Design review of the part shown in the three views and the two pictorial views. Dimensions are in mm from the part's minimum x, y and z. A direction names the side the tool comes from. Give positions to 0.01 mm unless a question says otherwise; leave off trailing zeros. Write each loop counter-clockwise with the first axis right and the second up, starting at its lowest first coordinate (ties: lowest second). Pieces come first, ordered by that corner, then holes. Notation, with made-up numbers: M 11,21.25 L 36,21.25 A25 cw 36,52.25 Z; hole C 71,-36.75 d10. An arc over 180 degrees is marked long. Use one line per item in the form item = value. Start each with the question number.
Q1. Consider section D-D on x = 13.5. Write out the cut boundary in (y, z), and give its area (3 significant figures).
Q2. Consider section B-B on z = 3.35. Write out the cut boundary in (x, y), and give its area (4 significant figures).
Q3. For probe 1 along X at (y, z) = (2.5, 1.2); probe 2 along Y at (x, z) = (16.5, 3.8), list the stretches that pass through material, from the lowest coordinate up. Write a range as [from, to].
Q4. Consider section C-C on y = 17.5. Write out the cut boundary in (x, z).
Q5. Consider section A-A on x = 3.75. Write out the cut boundary in (y, z), and give its area (3 significant figures).
Q6. Mouldability with a two-part tool opening along X and no side actions: class the marked faces 1, 2 and 3 as released by +X, released by -X, zero draft, split by the parting line, or undercut.
Q7. Clearance check with flat-ended pins moving along their axes: pin 1 Ø2 at (y, z) = (2.5, 2.5) entering from -X; pin 2 Ø2.5 at (x, z) = (2.5, 2.5) entering from -Y; pin 3 Ø8 at (x, y) = (8, 9) entering from -Z. State where each tip first meets the part, or that it passes through.
Q8. Tool access review of the marked faces 4, 5, 6 and 7: name each direction out of +Z, -Z, +X, -X, +Y, -Y from which nothing blocks a thin tool from reaching the whole face with its end or side.
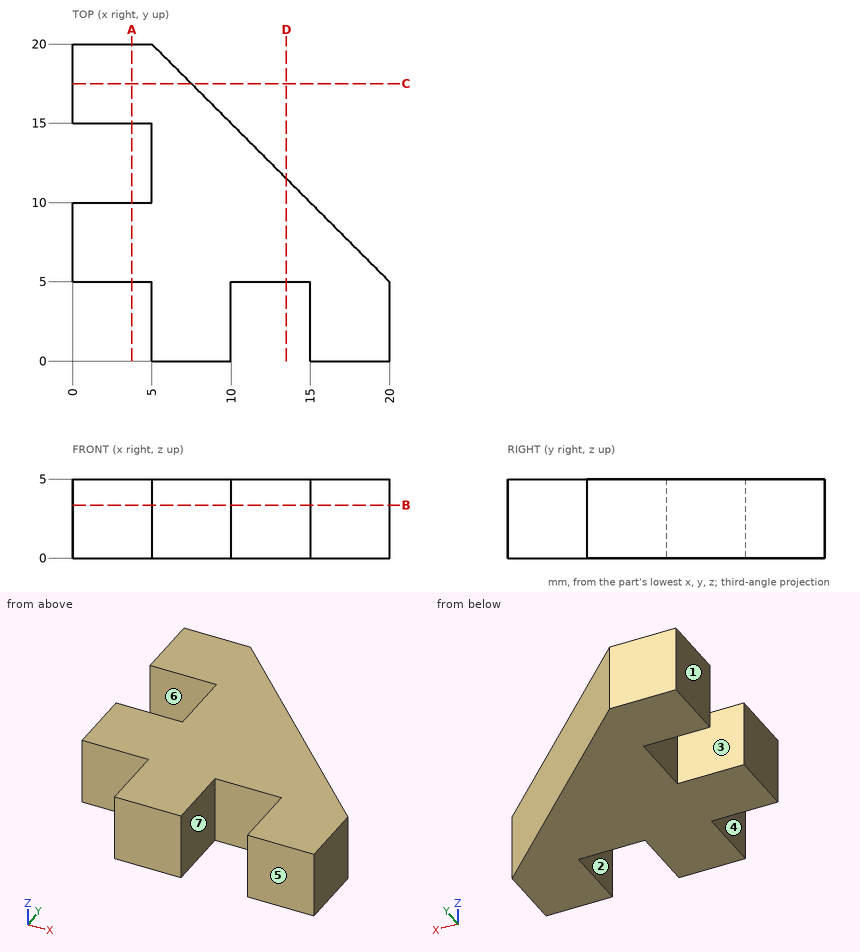
Working result:
q1.outline = M 5,0 L 11.5,0 L 11.5,5 L 5,5 Z
q1.area = 32.5 mm²
q2.outline = M 0,5 L 5,5 L 5,0 L 10,0 L 10,5 L 15,5 L 15,0 L 20,0 L 20,5 L 5,20 L 0,20 L 0,15 L 5,15 L 5,10 L 0,10 Z
q2.area = 212.5 mm²
q3.probe_1 = [5, 10], [15, 20]
q3.probe_2 = [0, 8.5]
q4.outline = M 0,0 L 7.5,0 L 7.5,5 L 0,5 Z
q5.outline = M 5,0 L 10,0 L 10,5 L 5,5 Z; M 15,0 L 20,0 L 20,5 L 15,5 Z
q5.area = 50.0 mm²
q6.face_1 = released by -X
q6.face_2 = undercut
q6.face_3 = zero draft
q7.pin_1 = 5
q7.pin_2 = 5
q7.pin_3 = 0
q8.face_4 = +Z, -Z, -X, -Y
q8.face_5 = +Z, -Z, +X, -X, -Y
q8.face_6 = +Z, -Z, -X
q8.face_7 = +Z, -Z, -Y
